Source: CAD feature listing. Evaluate the final solid. Frame: model axes, mm. Face numbers are marked on the shaded views. A direction names the side the tool comes from. Coordinates: 2 decimals unless noted, no trailing zeros. Order: outer loops, then holes, each group sorted by start corner. A loop starts at its lowest first (then second) coordinate and runs counter-clockwise, first axis right, second up.
```python
from build123d import *

# Parameters (mm, degrees)
SKIZZE1_W                            = 4
SKIZZE1_H                            = 4
AUFSATZ_LINEAR_AUSTRAGEN1_DEPTH      = 29.7
AUFSATZ_LINEAR_AUSTRAGEN2_DEPTH      = 0.2
AUFSATZ_LINEAR_AUSTRAGEN2_DEPTH_BACK = 4
AUFSATZ_LINEAR_AUSTRAGEN2_START      = 2
SKIZZE2_R                            = 2
SKIZZE3_R                            = 1
AUFSATZ_LINEAR_AUSTRAGEN4_DEPTH      = 4.5
VERRUNDUNG1_R                        = 2


with BuildPart() as part:
    # Skizze1 → Aufsatz-Linear austragen1 (new body)
    with BuildSketch(Plane.XY):
        Rectangle(SKIZZE1_W, SKIZZE1_H)
    extrude(amount=AUFSATZ_LINEAR_AUSTRAGEN1_DEPTH)

    # Skizze2 → Aufsatz-Linear austragen2 (add, two sides: drawn at the far end of the back side and taken through both)
    with BuildSketch(Plane(origin=(0, 0, 0), x_dir=(1, 0, 0), z_dir=(0, 1, 0)).offset(AUFSATZ_LINEAR_AUSTRAGEN2_START - AUFSATZ_LINEAR_AUSTRAGEN2_DEPTH_BACK)):
        with Locations(Location((0, -29.85, 0), (0, 0, 175.698777695))):
            Circle(SKIZZE2_R)
        with Locations(Location((0, 0.15, 0), (0, 0, 355.698777695))):
            Circle(SKIZZE2_R)
    extrude(amount=AUFSATZ_LINEAR_AUSTRAGEN2_DEPTH + AUFSATZ_LINEAR_AUSTRAGEN2_DEPTH_BACK)

    # Skizze3 → Aufsatz-Linear austragen4 (add)
    with BuildSketch(Plane(origin=(0, 2.2, 0), x_dir=(1, 0, 0), z_dir=(0, 1, 0))):
        with Locations(Location((0, -29.85, 0), (0, 0, 270))):
            Circle(SKIZZE3_R)
        with Locations(Location((0, 0.15, 0), (0, 0, 270))):
            Circle(SKIZZE3_R)
    extrude(amount=AUFSATZ_LINEAR_AUSTRAGEN4_DEPTH)

    # Verrundung1
    # the kernel refuses this fillet: 2 mm, written as the material it adds along each edge
    with BuildSketch(Plane(origin=(-1.994367068, 2, 29.7), x_dir=(-0.048500864171623644, 0, 0.9988231405882653), z_dir=(0, -1, 0)), Plane(origin=(1.994367068, 2, 0), x_dir=(0.04850086417162046, 0, -0.9988231405882655), z_dir=(0, -1, 0))) as verrundung1_piece_1:
        with BuildLine():
            CenterArc((0.159284835, 1.999295107), VERRUNDUNG1_R, 265.439839389, 3.038923762)
            Line((0.000273202, 0.005626303), (0, 0))
            ThreePointArc((0, 0), (0.053094945, 0.000704893), (0.10618989, 0))
        make_face()
    extrude(amount=4)
    with BuildSketch(Plane(origin=(1.994367068, -2, 29.7), x_dir=(1, 0, 0), z_dir=(0, 1, 0)), Plane(origin=(-1.994367068, -2, 0), x_dir=(-1, 0, 0), z_dir=(0, 1, 0))) as verrundung1_piece_2:
        with BuildLine():
            CenterArc((2.00466767, -0.062129838), VERRUNDUNG1_R, 178.219824845, 3.038923762)
            ThreePointArc((0.005150301, -0.106064919), (0.003279214, -0.052998272), (0, 0))
            Line((0, 0), (0.005632932, 0))
        make_face()
    extrude(amount=4)


solid = part.part
```
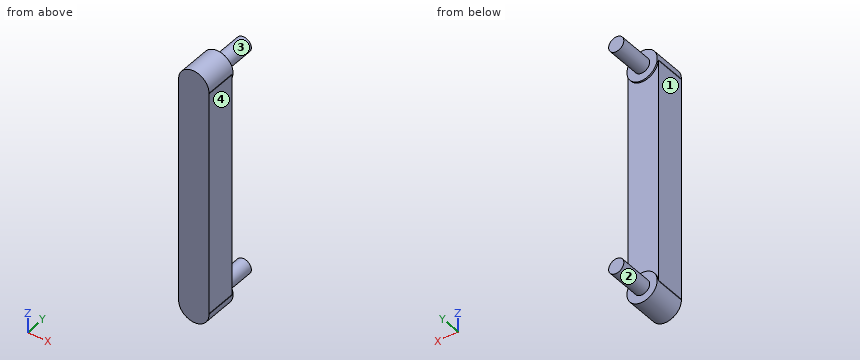
Q1. Section query C-C on y = -1. Output: boundary loops of the cut face in (x, z).
Solutions:
outline: (-2, -0.11) arc R2 ccw (long way) to (2, -0.11) arc R2 cw to (2, 0) - (2, 29.7) arc R2 cw to (2, 29.81) arc R2 ccw (long way) to (-2, 29.81) arc R2 cw to (-2, 29.7) - (-2, 0) arc R2 cw to start
Q2. Pin query (flat end, axial travel): P1, Ø1.2, axis at x = -0.5, z = 16.5, coming from the +Y side. Return the tip coordinate at first contact, or that it passes through.
Solutions:
P1: stops at y = 2
Q3. Section query D-D on z = 6.5. Output: boundary loops of the cut face in (x, y).
Solutions:
outline: (-2, -2) - (2, -2) - (2, 2) - (-2, 2) - close
Q4. Section query B-B on x = -0.5. Output: boundary loops of the cut face in (y, z), plus the area to 3 significant figures.
Solutions:
outline: (-2, -2.09) - (2.2, -2.09) - (2.2, -1.02) - (6.7, -1.02) - (6.7, 0.72) - (2.2, 0.72) - (2.2, 1.79) - (2, 1.79) - (2, 27.91) - (2.2, 27.91) - (2.2, 28.98) - (6.7, 28.98) - (6.7, 30.72) - (2.2, 30.72) - (2.2, 31.79) - (-2, 31.79) - close
area: 153 mm2
Q5. Pull-direction query (Z, two-part tool) for the marked faces 1 and 2; classes: pulls with the +Z half, pulls with the -Z half, needs draft (parallel to the pull), parting line crosses it, or undercut.
Solutions:
face 1: needs draft
face 2: undercut
Q6. Section query A-A on y = 2.5. Output: boundary loops of the cut face in (x, z).
Solutions:
outline: circle Ø2 at (0, -0.15); circle Ø2 at (0, 29.85)
Q7. Material intervals for line 1 along Y through (x, z) = (-0.1, 19); line 2 along Y through (x, z) = (-1.55, 29.5); line 3 along Z through (x, y) = (-0.85, 5), sorted ascending.
Solutions:
line 1: y = -2 to 2
line 2: y = -2 to 2.2
line 3: z = -0.68 to 0.38, 29.32 to 30.38
Q8. Set-up query: the marked faces 3 and 4. Return all of +Z, -Z, +X, -X, +Y, -Y with unobstructed straight access to the full face (end or side cutting, diameter ignored); none if empty.
Solutions:
face 3: +Y
face 4: +Z, -Z, +X, +Y, -Y
